Part model, mm, in its own coordinate system. A direction names the side the tool comes from. Coordinates: 2 decimals unless noted, no trailing zeros. Order: outer loops, then holes, each group sorted by start corner. A loop starts at its lowest first (then second) coordinate and runs counter-clockwise, first axis right, second up.
1) Tool access for faces 1 (the flat face through (-41, 4, 2)), 2 (the flat face through (-40, -4, 2)), 3 (the flat face through (-11.7, -2.2, 1)): list every direction of +Z, -Z, +X, -X, +Y, -Y with a clear straight run to the whole face (end or side of a thin tool).
2) Wall check: L1, parallel to Y at x = -12.5, z = 2.4; L2, parallel to X at y = -3.5, z = 1.3; L3, parallel to X at y = 3.75, z = 3.6. Give the ranges that are in metal, low to high.
3) Cut at B-B (x = -68). List the corners of the cut face in (y, z).
4) Cut at D-D (x = -37). List the corners of the cut face in (y, z), and give its area (3 significant figures).
5) Cut at A-A (z = 2.75). List the corners of the cut face in (x, y), and give its area (3 significant figures).
6) Mould opens along Y. For faces 4 (the flat face through (-67.7, -2.2, 1)), 5 (the cylindrical face through (-62.481, -4.255, 2.465)), 6 (the flat face through (-40, 0, 0)) say: +Y half, -Y half, draft (parallel to the pull), parting line (faces both ways), or undercut.
7) Pin check, flat tips, straight feed: pin 1 Ø1.5 at (x, z) = (-41, 2) entering from -Y; pin 2 Ø1.5 at (y, z) = (-4.5, 2.5) entering from +X; pin 3 Ø3.5 at (x, y) = (-70, -1) entering from +Z. Stop position of each tip, or through.
8) Cut at C-C (y = 0). Give the number of separate pieces and of enclosed holes in the cut face, and give its area (3 significant figures).
```python
from build123d import *

# Parameters (mm, degrees)
SKETCH1_R           = 1.75
BOSS_EXTRUDE1_DEPTH = 5
SKETCH2_R           = 7.25
BOSS_EXTRUDE2_DEPTH = 5
SKETCH5_R           = 5.95
CUT_EXTRUDE2_DEPTH  = 1
SKETCH6_R           = 2.25
CUT_EXTRUDE3_DEPTH  = 4
FILLET1_R           = 3
SKETCH7_R           = 5.2
CUT_EXTRUDE4_DEPTH  = 3


with BuildPart() as part:
    # Sketch1 → Boss-Extrude1 (new body)
    with BuildSketch(Plane.XY):
        with BuildLine():
            Line((-68.758315939, 4), (-12.748315939, 4))
            ThreePointArc((-12.748315939, 4), (-8.748315939, 0), (-12.748315939, -4))
            Line((-12.748315939, -4), (-68.758315939, -4))
            ThreePointArc((-68.758315939, -4), (-72.758315939, 0), (-68.758315939, 4))
        make_face()
        with Locations((-57.253315939, 0)):
            Circle(SKETCH1_R, mode=Mode.SUBTRACT)
        with Locations(Location((-24.253315939, 0, 0), (0, 0, 180))):
            Circle(SKETCH1_R, mode=Mode.SUBTRACT)
    extrude(amount=BOSS_EXTRUDE1_DEPTH)

    # Sketch2 → Boss-Extrude2 (add)
    with BuildSketch(Plane(origin=(0, 0, 0), x_dir=(-1, 0, 0), z_dir=(0, 0, -1))):
        with Locations((68.758315939, 0)):
            Circle(SKETCH2_R)
        with Locations((12.748315939, 0)):
            Circle(SKETCH2_R)
    extrude(amount=-BOSS_EXTRUDE2_DEPTH)

    # Sketch5 → Cut-Extrude2 (cut)
    with BuildSketch(Plane.XY.offset(5)):
        with Locations((-68.758315939, 0)):
            Circle(SKETCH5_R)
        with Locations((-12.748315939, 0)):
            Circle(SKETCH5_R)
    extrude(amount=-CUT_EXTRUDE2_DEPTH, mode=Mode.SUBTRACT)

    # Sketch6 → Cut-Extrude3 (cut)
    with BuildSketch(Plane(origin=(0, 0, 0), x_dir=(-1, 0, 0), z_dir=(0, 0, -1))):
        with Locations((12.748315939, 0)):
            Circle(SKETCH6_R)
        with Locations(Location((68.758315939, 0, 0), (0, 0, 180))):
            Circle(SKETCH6_R)
    extrude(amount=-CUT_EXTRUDE3_DEPTH, mode=Mode.SUBTRACT)

    # Fillet1
    fillet1_edges = [part.edges().sort_by_distance(p)[0] for p in [
        (-62.711622628, 4, 2.5),
        (-62.711622628, -4, 2.5),
        (-18.79500925, 4, 2.5),
        (-18.79500925, -4, 2.5),
    ]]
    fillet(fillet1_edges, radius=FILLET1_R)

    # Sketch7 → Cut-Extrude4 (cut)
    with BuildSketch(Plane.XY.offset(4)):
        with Locations((-68.758315939, 0)):
            Circle(SKETCH7_R)
        with Locations((-12.748315939, 0)):
            Circle(SKETCH7_R)
    extrude(amount=-CUT_EXTRUDE4_DEPTH, mode=Mode.SUBTRACT)


solid = part.part
```
Geometry check:
1. face 1: +Z, -Z, +Y
1. face 2: +Z, -Z, -Y
1. face 3: +Z
2. L1: y = -7.25 to -5.19, 5.19 to 7.25
2. L2: x = -75.11 to -72.6, -64.91 to -16.59, -8.9 to -6.4
2. L3: x = -74.96 to -72.36, -65.16 to -16.35, -9.15 to -6.54
3. outline: (-7.21, 0) - (-2.12, 0) - (-2.12, 1) - (-5.14, 1) - (-5.14, 4) - (-5.9, 4) - (-5.9, 5) - (-7.21, 5) - close; (2.12, 0) - (7.21, 0) - (7.21, 5) - (5.9, 5) - (5.9, 4) - (5.14, 4) - (5.14, 1) - (2.12, 1) - close
4. outline: (-4, 0) - (4, 0) - (4, 5) - (-4, 5) - close
4. area: 40.0 mm2
5. outline: (-63.46, -4.95) arc R3 cw to (-61.27, -4) - (-20.24, -4) arc R3 cw to (-18.04, -4.95) arc R7.25 ccw (long way) to (-18.04, 4.95) arc R3 cw to (-20.24, 4) - (-61.27, 4) arc R3 cw to (-63.46, 4.95) arc R7.25 ccw (long way) to start; hole circle Ø10.4 at (-68.76, 0); hole circle Ø3.5 at (-57.25, 0); hole circle Ø3.5 at (-24.25, 0); hole circle Ø10.4 at (-12.75, 0)
5. area: 480 mm2
6. face 4: undercut
6. face 5: -Y half
6. face 6: draft
7. pin 1: stops at y = -4
7. pin 2: stops at x = -6.54
7. pin 3: stops at z = 1
8. separate pieces: 5
8. enclosed holes: 0
8. area: 222 mm2
